Build history of the part. All positions in model axes, mm. Face numbers are marked on the shaded views. Round coordinates to 2 decimals unless told otherwise and drop trailing zeros. Loops run counter-clockwise (first coordinate to the right, second up) from the corner with the lowest first, then second, coordinate; pieces in that order, holes last. Notation, with made-up numbers: (14.25, -5) - (18.25, -5) arc R26 ccw to (18.25, 10) - close; hole circle Ø11 at (0.25, 32). An arc over 180 degrees is marked (long way). Use one line per item in the form item = value. Start each with the question number.
Q1. Saw through at A-A (y = 25.75). Give the cut face in (x, z), then the cut area to 3 significant figures.
Q2. Saw through at C-C (x = 0). Give the cut face in (y, z).
Q3. Drill centre lines: line 1 (Y direction, x = -58, z = -26); line 2 (X direction, y = 18.5, z = 28.5); line 3 (X direction, y = 25.5, z = 50.5). Where is each one in solid material? Low to high.
Q4. Mould opens along Z. For the marked faces 1, 2, 3 and 4 say: released by +Z, released by -Z, zero draft, split by the parting line, or undercut.
Q5. Pin check, flat tips, straight feed: pin 1 (1.1 mm diameter, centred on x = -9, y = 13.5, fed in from -Z); pin 2 (6 mm diameter, centred on x = -42, y = 20.5, fed in from +Z); pin 3 (1.5 mm diameter, centred on y = 1.5, z = -21, fed in from +X); pin 4 (6 mm diameter, centred on x = -2.5, z = -15, fed in from -Y). Stop position of each tip, or through.
Q6. Saw through at D-D (z = 45.5). Give the cut face in (x, y).
Q7. Saw through at B-B (z = -15.5). Give the cut face in (x, y), then the cut area to 3 significant figures.
Autodesk Inventor part; units mm, degrees
ref_plane "YZ Plane" through (0, 0, 0) normal (1, 0, 0) x (0, 1, 0)
ref_plane "XZ Plane" through (0, 0, 0) normal (0, 1, 0) x (-1, 0, 0)
ref_plane "XY Plane" through (0, 0, 0) normal (0, 0, 1) x (1, 0, 0)
sketch "Sketch1" plane through (0, 0, 0) normal (0, 1, 0) x (-1, 0, 0)
  circle A0 centre (0, 0) radius 70
  dimension "d0" = 140
extrude "Extrusion1" add sketch "Sketch1" along normal blind 28
sketch "Sketch2" plane through (0, 28, 0) normal (0, 1, 0) x (1, 0, 0)
  circle A0 centre (0, 0) radius 8.25
  dimension "d3" = 16.5
extrude "Extrusion2" cut sketch "Sketch2" against normal blind 28
sketch "Sketch3" plane through (0, 28, 0) normal (0, 1, 0) x (1, 0, 0)
  circle A0 centre (0, 0) radius 8.25
  circle A1 centre (0, 0) radius 65
  circle A2 centre (0, 0) radius 10.5
  dimension "d6" = 130
  dimension "d7" = 21
extrude "Extrusion3" cut sketch "Sketch3" against normal blind 25 contours A1
sketch "Sketch4" plane through (0, 3, 0) normal (0, 1, 0) x (1, 0, 0)
  line L0 (-77.4845, 0) -> (88.5537, 0)
  line L1 (88.5537, 0) -> (88.5537, 100.8261)
  line L2 (88.5537, 100.8261) -> (-77.4845, 100.8261)
  line L3 (-77.4845, 100.8261) -> (-77.4845, 0)
  point P0 (0, 0)
  point P1 (0, 0)
extrude "Extrusion4" cut sketch "Sketch4" along normal blind 220
sketch "Sketch5" plane through (0, 3, 0) normal (0, 1, 0) x (1, 0, 0)
  arc A0 (-10.5, 0) -> (10.5, 0) centre (0, 0) ccw
  arc A1 (-65, 0) -> (65, 0) centre (0, 0) ccw
  arc A2 (-10.5, 0) -> (10.5, 0) centre (0, 0) ccw
  line L0 (10.5, 0) -> (10.5, -64.1463)
  line L1 (-10.5, 0) -> (-10.5, -64.1463)
  arc A3 (-10.5, -64.1463) -> (10.5, -64.1463) centre (0, 0) ccw
  arc A4 (-10.5, 0) -> (10.5, 0) centre (0, 0) ccw
extrude "Extrusion5" add sketch "Sketch5" along normal blind 3
sketch "Sketch6" plane through (0, 28, 0) normal (0, 1, 0) x (1, 0, 0)
  line L0 (-8.25, 0) -> (-10.5, 0)
  line L1 (-8.25, 0) -> (8.25, 0)
  line L2 (8.25, 0) -> (8.25, 75.2128)
  line L3 (8.25, 75.2128) -> (-8.25, 75.2128)
  line L4 (-8.25, 75.2128) -> (-8.25, 0)
  point P0 (0, 0)
  dimension "d14" = 16.5
extrude "Extrusion6" cut sketch "Sketch6" against normal blind 30
sketch "Sketch8" plane through (0, 3, 0) normal (0, 1, 0) x (1, 0, 0)
  arc A0 (-65, 0) -> (65, 0) centre (0, 0) ccw
  line L0 (65, 0) -> (70, 0)
  arc A1 (70, 0) -> (-70, 0) centre (0, 0) ccw
  line L1 (-70, 0) -> (-65, 0)
  arc A2 (-10.5, 0) -> (10.5, 0) centre (0, 0) ccw
  line L2 (-10.5, 0) -> (-8.25, 0)
  arc A3 (8.25, 0) -> (-8.25, 0) centre (0, 0) ccw
  line L3 (8.25, 0) -> (10.5, 0)
  circle A4 centre (0, 0) radius 8.25
  arc A5 (65, 0) -> (-65, 0) centre (0, 0) ccw
  line L4 (-65, 0) -> (-70, 0)
  line L5 (65, 0) -> (70, 0)
  arc A6 (70, 0) -> (-70, 0) centre (0, 0) ccw
  arc A7 (70, 0) -> (70, 0) centre (0, 0) ccw
extrude "Extrusion7" cut sketch "Sketch8" against normal blind 30 contours L1 A1 L0 A5
properties part number "casept2"
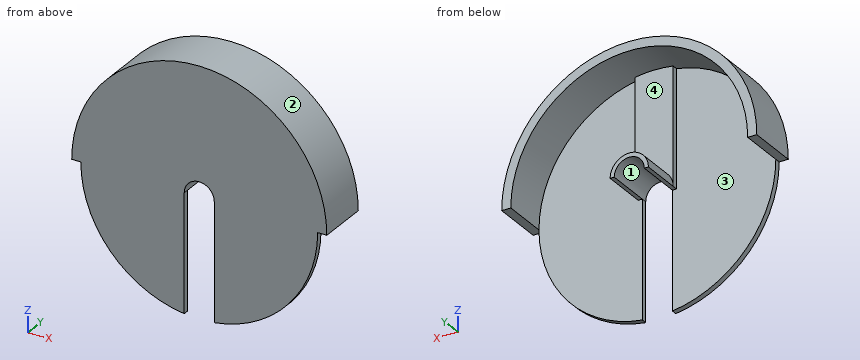
Report:
q1.outline = (-70, 0) - (-65, 0) arc R65 cw to (65, 0) - (70, 0) arc R70 ccw to start; (-10.5, 0) - (-8.25, 0) arc R8.25 cw to (8.25, 0) - (10.5, 0) arc R10.5 ccw to start
q1.area = 1,130 mm²
q2.outline = (0, 8.25) - (28, 8.25) - (28, 10.5) - (6, 10.5) - (6, 65) - (28, 65) - (28, 70) - (0, 70) - close
q3.line_1 = 0 to 3
q3.line_2 = -63.94 to -58.42, 58.42 to 63.94
q3.line_3 = -48.47 to -40.92, 40.92 to 48.47
q4.face_1 = released by -Z
q4.face_2 = released by +Z
q4.face_3 = zero draft
q4.face_4 = undercut
q5.pin_1 = 0
q5.pin_2 = 58.13
q5.pin_3 = 61.77
q5.pin_4 = through
q6.outline = (-53.2, 0) - (53.2, 0) - (53.2, 28) - (46.42, 28) - (46.42, 3) - (10.5, 3) - (10.5, 6) - (-10.5, 6) - (-10.5, 3) - (-46.42, 3) - (-46.42, 28) - (-53.2, 28) - close
q7.outline = (-63.12, 0) - (-8.25, 0) - (-8.25, 3) - (-63.12, 3) - close; (8.25, 0) - (63.12, 0) - (63.12, 3) - (8.25, 3) - close
q7.area = 329 mm²
